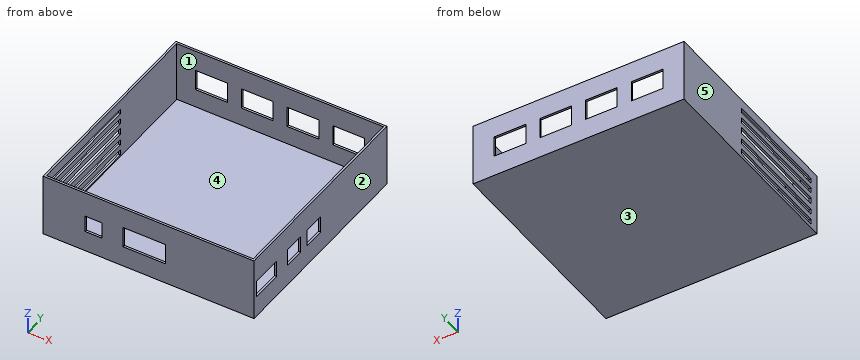
from build123d import *

# Parameters (mm, degrees)
F0_W      = 254
F0_H      = 254
F1_DEPTH  = 76.2
F2_W      = 248.92
F2_H      = 248.92
F3_DEPTH  = 73.66
F4_W      = 38.1
F4_H      = 25.4
F5_DEPTH  = 25.4
F6_W      = 38.1
F6_H      = 20.575085
F6_W_2    = 25.4
F7_DEPTH  = 25.4
F8_W      = 20.32
F8_H      = 20.32
F8_W_2    = 50.8
F8_H_2    = 25.4
F9_DEPTH  = 25.4
F10_W     = 132.736489
F10_H     = 6.033477
F10_H_2   = 6.512225
F10_H_3   = 7.788459
F10_H_4   = 6.512222
F10_H_5   = 6.788271
F11_DEPTH = 25.4


with BuildPart() as f1:
    # F0 (on Top) → F1 (new body)
    with BuildSketch(Plane.XY):
        with Locations((127, 127)):
            Rectangle(F0_W, F0_H)
    extrude(amount=F1_DEPTH)

    # F2 (on face) → F3 (cut)
    with BuildSketch(Plane.XY.offset(76.2)):
        with Locations((127, 127)):
            Rectangle(F2_W, F2_H)
    extrude(amount=-F3_DEPTH, mode=Mode.SUBTRACT)

    # F4 (on face) → F5 (cut)
    with BuildSketch(Plane(origin=(0, 254, 0), x_dir=(-1, 0, 0), z_dir=(0, 1, 0))):
        with Locations((-209.4992, 38.1)):
            Rectangle(F4_W, F4_H)
        with Locations((-154.4828, 38.1)):
            Rectangle(F4_W, F4_H)
        with Locations((-99.4664, 38.1)):
            Rectangle(F4_W, F4_H)
        with Locations((-44.45, 38.1)):
            Rectangle(F4_W, F4_H)
    extrude(amount=-F5_DEPTH, mode=Mode.SUBTRACT)

    # F6 (on face) → F7 (cut)
    with BuildSketch(Plane.YZ.offset(254)):
        with Locations((24.13, 35.687542)):
            Rectangle(F6_W, F6_H)
        with Locations((76.2, 35.687542)):
            Rectangle(F6_W_2, F6_H)
        with Locations((114.3, 35.687542)):
            Rectangle(F6_W_2, F6_H)
    extrude(amount=-F7_DEPTH, mode=Mode.SUBTRACT)

    # F8 (on face) → F9 (cut)
    with BuildSketch(Plane.XZ):
        with Locations((60.96, 35.56)):
            Rectangle(F8_W, F8_H)
        with Locations((121.92, 38.1)):
            Rectangle(F8_W_2, F8_H_2)
    extrude(amount=-F9_DEPTH, mode=Mode.SUBTRACT)

    # F10 (on face) → F11 (cut)
    with BuildSketch(Plane(origin=(0, 0, 0), x_dir=(0, -1, 0), z_dir=(-1, 0, 0))):
        with Locations((-77.526577, 61.941588)):
            Rectangle(F10_W, F10_H)
        with Locations((-77.526577, 49.178708)):
            Rectangle(F10_W, F10_H_2)
        with Locations((-77.526577, 35.516145)):
            Rectangle(F10_W, F10_H_3)
        with Locations((-77.526577, 21.126057)):
            Rectangle(F10_W, F10_H_4)
        with Locations((-77.526577, 7.713118)):
            Rectangle(F10_W, F10_H_5)
    extrude(amount=-F11_DEPTH, mode=Mode.SUBTRACT)


solid = f1.part
Could you check a few things on this model? Use its own coordinates, in mm. Face numbers are marked on the shaded views. A direction names the side the tool comes from. Give positions to 0.01 mm unless a question says otherwise; leave off trailing zeros. Loops run counter-clockwise (first coordinate to the right, second up) from the corner with the lowest first, then second, coordinate; pieces in that order, holes last. Notation, with made-up numbers: (1, 9.25) -> (40, 9.25) arc R17 ccw to (40, 28.25) -> close; hole circle Ø10 at (48, 5). An arc over 180 degrees is marked (long way). Answer as CSV lines item,"result". Start each with the question number.
(1) If we section it at A-A on y = 69: Count the separate pieces of the cut face and the enclosed holes in it, then the cut area to 3 significant figures.
(2) We'd pull the mould along X, two halves only. Please class the marked faces 3, 4 and 5: released by +X, released by -X, zero draft, split by the parting line, or undercut.
(3) I need wall thicknesses on probe 1 along Y at (x, z) = (99.5, 61.5); probe 2 along Z at (x, y) = (155.5, 214). Which ranges of each line are inside material? Lowest first, please.
(4) If we section it at B-B on x = 109: Write out the boundary of the cut face in (y, z).
(5) If we section it at C-C on x = 214.5: Write out the boundary of the cut face in (y, z).
(6) If we section it at D-D on z = 55.5: Write out the boundary of the cut face in (x, y).
(7) Which directions (+Z, -Z, +X, -X, +Y, -Y) give clear straight access to the entire face, cutting with the end or side of a thin tool? Please do the marked faces 1 and 2.
(8) I'm going to push flat-ended pins straight in: pin 1 Ø12 at (x, z) = (62, 42.5) entering from -Y; pin 2 Ø1.5 at (x, y) = (115, 195.5) entering from +Z. Where does each tip first touch, or does it pass through?
Computed:
1,separate pieces,"7"
1,enclosed holes,"0"
1,area,"882 mm2"
2,face 3,"zero draft"
2,face 4,"undercut"
2,face 5,"released by -X"
3,probe 1,"y = 0 to 2.54, 251.46 to 254"
3,probe 2,"z = 0 to 2.54"
4,outline,"(0, 0) -> (254, 0) -> (254, 25.4) -> (251.46, 25.4) -> (251.46, 2.54) -> (2.54, 2.54) -> (2.54, 25.4) -> (0, 25.4) -> close; (0, 50.8) -> (2.54, 50.8) -> (2.54, 76.2) -> (0, 76.2) -> close; (251.46, 50.8) -> (254, 50.8) -> (254, 76.2) -> (251.46, 76.2) -> close"
5,outline,"(0, 0) -> (254, 0) -> (254, 25.4) -> (251.46, 25.4) -> (251.46, 2.54) -> (2.54, 2.54) -> (2.54, 76.2) -> (0, 76.2) -> close; (251.46, 50.8) -> (254, 50.8) -> (254, 76.2) -> (251.46, 76.2) -> close"
6,outline,"(0, 0) -> (254, 0) -> (254, 254) -> (0, 254) -> close; hole (2.54, 2.54) -> (251.46, 2.54) -> (251.46, 251.46) -> (2.54, 251.46) -> close"
7,face 1,"+Z"
7,face 2,"+Z, -Z, +X, +Y, -Y"
8,pin 1,"stops at y = 0"
8,pin 2,"stops at z = 2.54"
